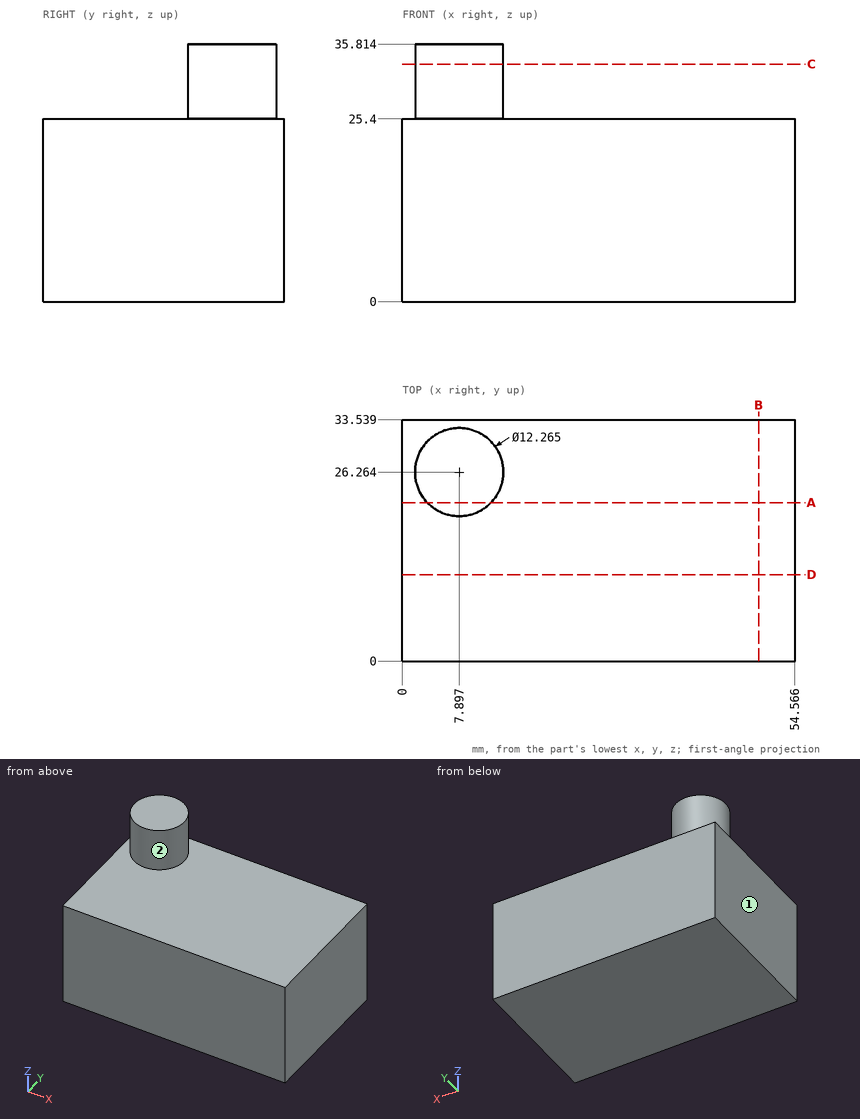
Here's the drawing with two shaded views (mm, measured from the low corner). I have some questions. A direction names the side the tool comes from. Coordinates: 2 decimals unless noted, no trailing zeros. Loops run counter-clockwise (first coordinate to the right, second up) from the corner with the lowest first, then second, coordinate; pieces in that order, holes last.
Item 1: Which directions (+Z, -Z, +X, -X, +Y, -Y) give clear straight access to the entire face, cutting with the end or side of a thin tool? Please do the marked faces 1 and 2.
Answers below:
face 1: +Z, -Z, -X, +Y, -Y
face 2: +Z
Item 2: Please list where these lines run through material, in increasing order: L1, parallel to Z at x = 39.5, y = 29; L2, parallel to Y at x = 9, z = 32.5; L3, parallel to Y at x = 4, z = 28.5.
Answers below:
L1: z = 0 to 25.4
L2: y = 20.23 to 32.3
L3: y = 21.53 to 31
Item 3: Suppose I cut it at B-B (x = 49.5). Please give me the cut outline in (y, z).
Answers below:
outline: (0, 0) - (33.54, 0) - (33.54, 25.4) - (0, 25.4) - close
Item 4: Suppose I cut it at A-A (y = 22). Please give me the cut outline in (x, z) (1 decimal).
Answers below:
outline: (0, 0) - (54.6, 0) - (54.6, 25.4) - (12.3, 25.4) - (12.3, 35.8) - (3.5, 35.8) - (3.5, 25.4) - (0, 25.4) - close
Item 5: Suppose I cut it at C-C (z = 33). Please give me the cut outline in (x, y) (1 decimal), then the cut area to 3 significant figures.
Answers below:
outline: circle Ø12.3 at (7.9, 26.3)
area: 118 mm2
Item 6: I'm going to push flat-ended pins straight in: pin 1 (12 mm diameter, centred on x = 47.5, z = 12.5, fed in from -Y); pin 2 (4 mm diameter, centred on x = 38.5, y = 12, fed in from +Z). Where does each tip first touch, or does it pass through?
Answers below:
pin 1: stops at y = 0
pin 2: stops at z = 25.4
Item 7: Suppose I cut it at D-D (y = 12). Please give me the cut outline in (x, z), then the cut area to 3 significant figures.
Answers below:
outline: (0, 0) - (54.57, 0) - (54.57, 25.4) - (0, 25.4) - close
area: 1,390 mm2
